Geometry check sheet. Reference: the model listing, model coordinates, mm. Coordinates: 2 decimals unless noted, no trailing zeros. Order: outer loops, then holes, each group sorted by start corner. A loop starts at its lowest first (then second) coordinate and runs counter-clockwise, first axis right, second up. Notation, with made-up numbers: (-39.75, 9) -> (-18.75, 9) arc R22 cw to (-18.75, 17) -> close; hole circle Ø1 at (11, -19). An arc over 180 degrees is marked (long way). Answer in a Markdown table with one row per item. Add a question column.
```python
from build123d import *

# Parameters (mm, degrees)
EXTRUDE1_DEPTH = 0.8128
FILLET1_R      = 2.54


with BuildPart() as part:
    # Sketch1 → Extrude1 (new body)
    with BuildSketch(Plane(origin=(0, 0, 0), x_dir=(1, 0, 0), z_dir=(0, 1, 0))):
        Polygon((-30.576142977, 61.517339059), (-63.530339059, 28.563142977), (-63.530339059, -28.563142977), (-30.576142977, -61.517339059), (30.576142977, -61.517339059), (63.530339059, -28.563142977), (63.530339059, 28.563142977), (30.576142977, 61.517339059), align=None)
    extrude(amount=EXTRUDE1_DEPTH)

    # Fillet1
    fillet1_edges = [part.edges().sort_by_distance(p)[0] for p in [
        (30.576142977, 0.4064, -61.517339059),
        (63.530339059, 0.4064, -28.563142977),
        (63.530339059, 0.4064, 28.563142977),
        (30.576142977, 0.4064, 61.517339059),
        (-30.576142977, 0.4064, 61.517339059),
        (-63.530339059, 0.4064, 28.563142977),
        (-63.530339059, 0.4064, -28.563142977),
        (-30.576142977, 0.4064, -61.517339059),
    ]]
    fillet(fillet1_edges, radius=FILLET1_R)


solid = part.part
```
(1) Scan lines: line 1 along Z through (x, y) = (-57.5, 0.4); line 2 along X through (y, z) = (0.1, -31.5); line 3 along X through (y, z) = (0.2, -34). Record each from-to range of solid material in increasing order.
(2) Cross-section at C-C (x = -49.5). Enter the section's corners in (y, z), plus the area to 3 significant figures.
(3) Cross-section at A-A (y = 0.4). Enter the section's corners in (x, z), plus the area to 3 significant figures.
(4) Mould release check, pull along Z, two halves, no side actions. Record for faces 1 (the face through (-47.274, 0.401, 44.82)), 2 (the face through (-46.833, 0.401, -45.261)), 3 (the face through (-1, 0, -1)): +Z half, -Z half, draft (parallel to the pull), parting line (faces both ways), or undercut.
(5) Cross-section at B-B (z = 43). Enter the section's corners in (x, y).
Checks:
| question | item | result |
|---|---|---|
| 1 | line 1 | -34.59 to 34.59 |
| 1 | line 2 | -60.59 to 60.59 |
| 1 | line 3 | -58.09 to 58.09 |
| 2 | outline | (0, -42.59) -> (0.81, -42.59) -> (0.81, 42.59) -> (0, 42.59) -> close |
| 2 | area | 69.2 mm² |
| 3 | outline | (-63.53, -27.51) arc R2.54 ccw to (-62.79, -29.31) -> (-31.32, -60.77) arc R2.54 ccw to (-29.52, -61.52) -> (29.52, -61.52) arc R2.54 ccw to (31.32, -60.77) -> (62.79, -29.31) arc R2.54 ccw to (63.53, -27.51) -> (63.53, 27.51) arc R2.54 ccw to (62.79, 29.31) -> (31.32, 60.77) arc R2.54 ccw to (29.52, 61.52) -> (-29.52, 61.52) arc R2.54 ccw to (-31.32, 60.77) -> (-62.79, 29.31) arc R2.54 ccw to (-63.53, 27.51) -> close |
| 3 | area | 13,500 mm² |
| 4 | face 1 | +Z half |
| 4 | face 2 | -Z half |
| 4 | face 3 | draft |
| 5 | outline | (-49.09, 0) -> (49.09, 0) -> (49.09, 0.81) -> (-49.09, 0.81) -> close |
